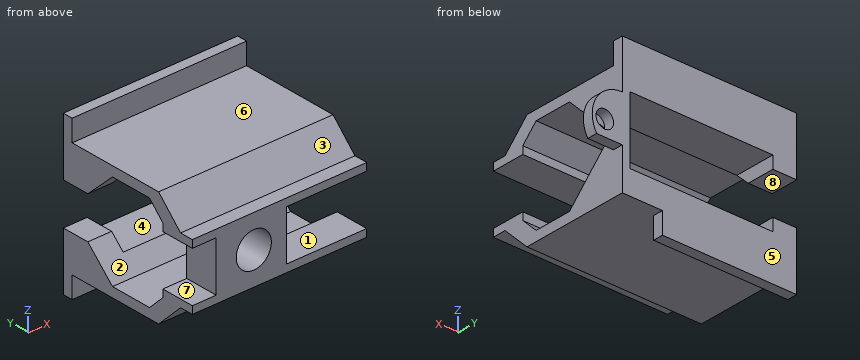
Autodesk Fusion 360 part; units mm, degrees
sketch "Sketch1" plane through (0, 0, 0) normal (0, 1, 0) x (1, 0, 0)
  line L0 (0, 0) -> (0, 11.5)
  line L1 (0, 0) -> (0, -8.3) construction
  line L2 (0, -8.3) -> (0, -19.8)
  line L3 (0, -19.8) -> (34.75, -19.8)
  line L4 (34.75, -19.8) -> (34.75, -10.025)
  line L5 (0, 11.5) -> (26.75, 11.5)
  line L6 (26.75, 11.5) -> (26.75, 7.25)
  line L7 (26.75, 7.25) -> (34.75, 7.25)
  line L8 (34.75, 7.25) -> (34.75, 1.85)
  line L9 (0, 0) -> (4.75, 0)
  line L10 (0, -8.3) -> (4.75, -8.3)
  line L11 (4.75, 0) -> (4.75, 2.475)
  line L12 (4.75, 2.475) -> (33.25, 2.475)
  line L13 (4.75, -8.3) -> (4.75, -10.775)
  line L14 (4.75, -10.775) -> (33.25, -10.775)
  line L15 (33.25, -10.775) -> (33.25, 2.475)
  line L16 (33.25, -4.15) -> (34.75, -4.15)
  arc A0 (34.75, -10.15) -> (34.75, 1.85) centre (34.75, -4.15) ccw
  line L17 (33.25, -4.15) -> (38.25, -4.15)
  circle A1 centre (38.25, -4.15) radius 1.75
  dimension "d1" = 11.5
  dimension "d2" = 8.3
  dimension "d3" = 11.5
  dimension "d4" = 34.75
  dimension "d5" = 9.775
  dimension "d6" = 26.75
  dimension "d7" = 4.25
  dimension "d8" = 8
  dimension "d10" = 4.75
  dimension "d11" = 4.75
  dimension "d12" = 2.475
  dimension "d13" = 28.5
  dimension "d14" = 2.475
  dimension "d15" = 28.5
  dimension "d16" = 12
  dimension "d17" = 5
  dimension "d18" = 3.5
extrude "Extrude1" add sketch "Sketch1" against normal blind 2
sketch "Sketch2" plane through (0, 0, 0) normal (-1, 0, 0) x (0, 0, 1)
  line L0 (0, 0) -> (-11.5, 0)
  line L1 (-11.5, 0) -> (-11.5, -2)
  line L2 (-11.5, -2) -> (0, -2)
  line L3 (0, -2) -> (0, 0)
  line L4 (0, -2) -> (0, -5.535)
  line L5 (8.3, -2) -> (8.3, -5.535)
  line L6 (0, -2) -> (-7.25, -2) construction
  line L7 (8.3, -2) -> (15.55, -2) construction
  line L8 (-7.25, -2) -> (-7.25, -21.5)
  line L9 (15.55, -2) -> (15.55, -21.5)
  line L10 (-7.25, -21.5) -> (-2.3003, -26.4497)
  line L11 (-7.25, -21.5) -> (-0.25, -21.5) construction
  line L12 (15.55, -21.5) -> (10.6003, -26.4497)
  line L13 (15.55, -21.5) -> (22.55, -21.5) construction
  line L14 (-2.3003, -26.4497) -> (-2.3003, -29.5997)
  line L15 (10.6003, -26.4497) -> (10.6003, -29.5997)
  line L16 (-2.3003, -29.5997) -> (10.6003, -29.5997)
  line L17 (-2.3003, -29.5997) -> (-2.3003, -22.4497) construction
  line L18 (10.6003, -29.5997) -> (10.6003, -22.4497) construction
  line L19 (10.6003, -22.4497) -> (-2.3003, -22.4497)
  line L20 (-2.3003, -22.4497) -> (-5.3055, -19.4445)
  line L21 (-2.3003, -22.4497) -> (1.9497, -22.4497) construction
  line L22 (10.6003, -22.4497) -> (13.6055, -19.4445)
  line L23 (10.6003, -22.4497) -> (14.8503, -22.4497) construction
  line L24 (-5.3055, -19.4445) -> (-5.3055, -11.0945)
  line L25 (13.6055, -19.4445) -> (13.6055, -11.0945)
  line L26 (-5.3055, -11.0945) -> (0, -5.535)
  line L27 (13.6055, -11.0945) -> (8.3, -5.535)
  line L28 (-7.25, -2) -> (0, -2)
  line L29 (8.3, -2) -> (15.55, -2)
  point P0 (8.3, -2)
  dimension "d24" = 3.535
  dimension "d25" = 3.535
  dimension "d26" = 7.25
  dimension "d27" = 7.25
  dimension "d28" = 19.5
  dimension "d29" = 19.5
  dimension "d30" = 45
  dimension "d31" = 7
  dimension "d32" = 135
  dimension "d33" = 7
  dimension "d34" = 3.15
  dimension "d35" = 3.15
  dimension "d36" = 7.15
  dimension "d37" = 7.15
  dimension "d38" = 135
  dimension "d39" = 4.25
  dimension "d40" = 45
  dimension "d41" = 4.25
  dimension "d42" = 8.35
  dimension "d43" = 8.35
extrude "Extrude2" add sketch "Sketch2" against normal blind 34.75 contours L2 L4 L5 L8 L9 L10 L12 L14 L15 L16 L19 L20 L22 L24 L25 L26 L27 L28 L29
extrude "Extrude3" cut 2 faces at (14.25, -2, -1.65) (23.75, -2, 9.125) along direction (0, -1, 0) blind 10
sketch "Sketch3" plane through (0, 0, 0) normal (0, 1, 0) x (-1, 0, 0)
  circle A0 centre (-38.25, 4.15) radius 1.75
  line L0 (0, 8.3) -> (0, 19.8)
  line L1 (0, 19.8) -> (-34.75, 19.8)
  line L2 (-34.75, 19.8) -> (-34.75, 10.15)
  arc A1 (-34.75, 10.15) -> (-34.75, -1.85) centre (-34.75, 4.15) ccw
  line L3 (-34.75, -1.85) -> (-34.75, -7.25)
  line L4 (-34.75, -7.25) -> (-26.75, -7.25)
  line L5 (-26.75, -7.25) -> (-26.75, -11.5)
  line L6 (-26.75, -11.5) -> (0, -11.5)
  line L7 (0, -11.5) -> (0, 0)
  line L8 (0, 0) -> (-4.75, 0)
  line L9 (-4.75, 0) -> (-4.75, -2.475)
  line L10 (-4.75, -2.475) -> (-33.25, -2.475)
  line L11 (-33.25, -2.475) -> (-33.25, 10.775)
  line L12 (-33.25, 10.775) -> (-4.75, 10.775)
  line L13 (-4.75, 10.775) -> (-4.75, 8.3)
  line L14 (-4.75, 8.3) -> (0, 8.3)
  line L15 (-34.75, -1.85) -> (-34.75, 1.025)
  line L16 (-34.75, 1.025) -> (-41.4539, 1.025)
  dimension "d48" = 2.875
extrude "Extrude4" cut sketch "Sketch3" against normal blind 13 contours A1 L15 L16
sketch "Sketch4" plane through (34.75, 0, 0) normal (1, 0, 0) x (0, 0, -1)
  line L0 (0, -5.535) -> (5.3055, -11.0945)
  line L1 (5.3055, -11.0945) -> (5.3055, -19.4445)
  line L2 (5.3055, -19.4445) -> (2.3003, -22.4497)
  line L3 (2.3003, -22.4497) -> (-10.6003, -22.4497)
  line L4 (-10.6003, -22.4497) -> (-13.6055, -19.4445)
  line L5 (-13.6055, -19.4445) -> (-13.6055, -11.0945)
  line L6 (-13.6055, -11.0945) -> (-8.3, -5.535)
  line L7 (-8.3, -5.535) -> (-8.3, -2)
  line L8 (-8.3, -2) -> (-10.15, -2)
  line L9 (-10.15, -2) -> (-10.15, 0)
  line L10 (-10.15, 0) -> (-19.8, 0)
  line L11 (-19.8, 0) -> (-19.8, -2)
  line L12 (-19.8, -2) -> (-15.55, -2)
  line L13 (-15.55, -2) -> (-15.55, -21.5)
  line L14 (-15.55, -21.5) -> (-10.6003, -26.4497)
  line L15 (-10.6003, -26.4497) -> (-10.6003, -29.5997)
  line L16 (-10.6003, -29.5997) -> (2.3003, -29.5997)
  line L17 (2.3003, -29.5997) -> (2.3003, -26.4497)
  line L18 (2.3003, -26.4497) -> (7.25, -21.5)
  line L19 (7.25, -21.5) -> (7.25, 0)
  line L20 (7.25, 0) -> (-1.025, 0)
  line L21 (-1.025, 0) -> (-1.025, -2)
  line L22 (-1.025, -2) -> (0, -2)
  line L23 (0, -2) -> (0, -5.535)
  line L24 (-3.535, -2) -> (-3.6055, -1.9295)
  line L25 (0, -5.535) -> (10, -5.535) construction
  line L26 (-4.765, -2) -> (-4.6945, -1.9295)
  line L27 (-8.3, -5.535) -> (1.7, -5.535) construction
  line L28 (-16, -15) -> (-15.5, -15)
  line L29 (-13.6055, -11.0945) -> (-13.6055, -11.9295)
  line L30 (-13.6055, -11.9295) -> (6.3945, -11.9295) construction
  line L31 (5.3055, -11.0945) -> (5.3055, -11.9295)
  line L32 (5.3055, -11.9295) -> (25.3055, -11.9295) construction
  line L33 (-8.3, -5.535) -> (-8.3, -2)
  line L34 (-8.3, -2) -> (0, -2)
  line L35 (0, -2) -> (0, -5.535)
  line L36 (0, -5.535) -> (5.3055, -11.0945)
  line L37 (-13.6055, -11.9295) -> (-4.15, -2.4741)
  line L38 (-3.6759, -2) -> (-3.6055, -1.9295)
  line L39 (5.3055, -11.9295) -> (-4.15, -2.4741)
  line L40 (-4.6241, -2) -> (-4.6945, -1.9295)
  dimension "d51" = 135
  dimension "d53" = 45
  dimension "d55" = 0.835
  dimension "d56" = 45
  dimension "d58" = 0.835
  dimension "d59" = 135
extrude "Extrude5" add sketch "Sketch4" against normal blind 1.5 contours L0 L1 L5 L6 L7 L22 L23 L29 L31 L33 L34 L35 L36 L37 L39
sketch "Sketch5" plane through (0, -29.5997, 0) normal (0, -1, 0) x (1, 0, 0)
  line L0 (0, 10.6003) -> (0, -2.3003)
  line L1 (0, -2.3003) -> (34.75, -2.3003)
  line L2 (34.75, -2.3003) -> (34.75, 10.6003)
  line L3 (34.75, 10.6003) -> (0, 10.6003)
  line L4 (0, 4.15) -> (12.25, 4.15)
  circle A0 centre (12.25, 4.15) radius 3.5
  dimension "d63" = 12.25
  dimension "d65" = 7
extrude "Extrude6" cut sketch "Sketch5" against normal blind 13 contours A0
sketch "Sketch6" plane through (34.75, 0, 0) normal (1, 0, 0) x (0, 0, -1)
  line L0 (-1.025, -2) -> (-10.15, -2)
  line L1 (-10.15, -2) -> (-10.15, 0)
  line L2 (-10.15, 0) -> (-19.8, 0)
  line L3 (-19.8, 0) -> (-19.8, -2)
  line L4 (-19.8, -2) -> (-15.55, -2)
  line L5 (-15.55, -2) -> (-15.55, -21.5)
  line L6 (-15.55, -21.5) -> (-10.6003, -26.4497)
  line L7 (-10.6003, -26.4497) -> (-10.6003, -29.5997)
  line L8 (-10.6003, -29.5997) -> (2.3003, -29.5997)
  line L9 (2.3003, -29.5997) -> (2.3003, -26.4497)
  line L10 (2.3003, -26.4497) -> (7.25, -21.5)
  line L11 (7.25, -21.5) -> (7.25, 0)
  line L12 (7.25, 0) -> (-1.025, 0)
  line L13 (-1.025, 0) -> (-1.025, -2)
  line L14 (-13.6055, -11.9295) -> (-4.15, -2.4741)
  line L15 (-4.15, -2.4741) -> (5.3055, -11.9295)
  line L16 (5.3055, -11.9295) -> (5.3055, -19.4445)
  line L17 (5.3055, -19.4445) -> (2.3003, -22.4497)
  line L18 (2.3003, -22.4497) -> (-10.6003, -22.4497)
  line L19 (-10.6003, -22.4497) -> (-13.6055, -19.4445)
  line L20 (-13.6055, -19.4445) -> (-13.6055, -11.9295)
  line L21 (2.3003, -29.5997) -> (0.8003, -29.5997)
  line L22 (-10.6003, -29.5997) -> (-9.1003, -29.5997)
  line L23 (-9.1003, -29.5997) -> (-9.1003, -22.4494)
  line L24 (0.8003, -29.5997) -> (0.8003, -22.4497)
  dimension "d69" = 1.5
  dimension "d70" = 1.5
  dimension "d71" = 7.15
extrude "Extrude7" cut sketch "Sketch6" against normal blind 16 contours L8 L18 L23 L24
sketch "Sketch7" plane through (0, 0, 0) normal (-1, 0, 0) x (0, 0, 1)
  line L0 (0, 0) -> (-11.5, 0)
  line L1 (-11.5, 0) -> (-11.5, -2)
  line L2 (-11.5, -2) -> (-7.25, -2)
  line L3 (-7.25, -2) -> (-7.25, -21.5)
  line L4 (-7.25, -21.5) -> (-2.3003, -26.4497)
  line L5 (-2.3003, -26.4497) -> (-2.3003, -29.5997)
  line L6 (-2.3003, -29.5997) -> (10.6003, -29.5997)
  line L7 (10.6003, -29.5997) -> (10.6003, -26.4497)
  line L8 (10.6003, -26.4497) -> (15.55, -21.5)
  line L9 (15.55, -21.5) -> (15.55, -2)
  line L10 (15.55, -2) -> (19.8, -2)
  line L11 (19.8, -2) -> (19.8, 0)
  line L12 (19.8, 0) -> (8.3, 0)
  line L13 (8.3, 0) -> (8.3, -5.535)
  line L14 (8.3, -5.535) -> (13.6055, -11.0945)
  line L15 (13.6055, -11.0945) -> (13.6055, -19.4445)
  line L16 (13.6055, -19.4445) -> (10.6003, -22.4497)
  line L17 (10.6003, -22.4497) -> (-2.3003, -22.4497)
  line L18 (-2.3003, -22.4497) -> (-5.3055, -19.4445)
  line L19 (-5.3055, -19.4445) -> (-5.3055, -11.0945)
  line L20 (-5.3055, -11.0945) -> (0, -5.535)
  line L21 (0, -5.535) -> (0, 0)
  line L22 (10.6003, -29.5997) -> (9.1003, -29.5997)
  line L23 (-2.3003, -29.5997) -> (-0.8003, -29.5997)
  line L24 (-0.8003, -29.5997) -> (-0.8003, -22.4497)
  line L25 (9.1003, -29.5997) -> (9.1003, -22.4497)
  point P0 (-0.8003, -22.4497)
  point P1 (9.1003, -22.4497)
  dimension "d74" = 1.5
  dimension "d75" = 1.5
extrude "Extrude8" cut sketch "Sketch7" against normal blind 4.75 contours L6 L17 L24 L25
extrude "Extrude9" cut 1 faces at (6.0833, -29.5997, 4.15) along direction (0, 1, 0) blind 0.5
sketch "Sketch8" plane through (0, 0, 0) normal (0, 1, 0) x (-1, 0, 0)
  line L0 (-39.872, 1.025) -> (-34.75, 1.025)
  line L1 (-34.75, 1.025) -> (-34.75, -7.25)
  line L2 (-34.75, -7.25) -> (-26.75, -7.25)
  line L3 (-26.75, -7.25) -> (-26.75, -11.5)
  line L4 (-26.75, -11.5) -> (0, -11.5)
  line L5 (0, -11.5) -> (0, 0)
  line L6 (0, 0) -> (-4.75, 0)
  line L7 (-4.75, 0) -> (-4.75, -2.475)
  line L8 (-4.75, -2.475) -> (-33.25, -2.475)
  line L9 (-33.25, -2.475) -> (-33.25, 10.775)
  line L10 (-33.25, 10.775) -> (-4.75, 10.775)
  line L11 (-4.75, 10.775) -> (-4.75, 8.3)
  line L12 (-4.75, 8.3) -> (0, 8.3)
  line L13 (0, 8.3) -> (0, 19.8)
  line L14 (0, 19.8) -> (-34.75, 19.8)
  line L15 (-34.75, 19.8) -> (-34.75, 10.15)
  arc A0 (-34.75, 10.15) -> (-39.872, 1.025) centre (-34.75, 4.15) ccw
  circle A1 centre (-38.25, 4.15) radius 1.75
  line L16 (-34.75, 10.15) -> (-34.75, 1.025)
  line L17 (-34.75, 4.15) -> (-38.25, 4.15)
equation "d17 = HolePosX"
equation "d18 = HoleSize"
equation "HolePosX = 5 mm"
equation "HoleSize = 3.5 mm"
equation "TopThickness = 2 mm"
equation "d63 = JointPosX"
equation "JointPosX = 12.25 mm"
equation "d65 = HoleBall"
equation "HoleBall = 7 mm"
Can you work these out from the model? Positions are in its coordinate system, mm. Face numbers are marked on the shaded views. A direction names the side the tool comes from. Coordinates: 2 decimals unless noted, no trailing zeros. Write each loop counter-clockwise with the first axis right and the second up, starting at its lowest first coordinate (ties: lowest second). Pieces come first, ordered by that corner, then holes. Notation, with made-up numbers: (39.5, 50) -> (63.5, 50) arc R14 cw to (63.5, 72) -> close; hole circle Ø6 at (53.5, 48). An arc over 180 degrees is marked (long way). Write each question's results on one line, items separated by ' | '. Start each with the question number.
Q1. Imagine slicing it at C-C (y = -9). Write out the boundary of the cut face in (x, z), then the cut area to 3 significant figures.
Q2. Imagine slicing it at D-D (z = 12). Write out the boundary of the cut face in (x, y), then the cut area to 3 significant figures.
Q3. On a 3-axis mill with a long thin cutter (end or side, diameter ignored), from which of +Z, -Z, +X, -X, +Y, -Y can I reach the whole of each face in a straight line? I mean the marked faces 4, 5, 6, 7 and 8. Say none if no direction works.
Q4. If I drill on probe 1 along Z at (x, y) = (7, -12); probe 2 along Z at (x, y) = (21, -5.5) (3 decimals); probe 3 along X at (y, z) = (-0.65, 4.15), over which ranges is the centre line in solid material (lowest first)?
Q5. Imagine slicing it at A-A (y = -23.25). Write out the boundary of the cut face in (x, z), then the cut area to 3 significant figures.
Q6. I'm going to push flat-ended pins straight in: pin 1 (8 mm diameter, centred on y = -19.5, z = -4.5, fed in from +X); pin 2 (6.5 mm diameter, centred on x = 15.5, y = -16.5, fed in from +Z); pin 3 (2 mm diameter, centred on x = 26, z = 18.5, fed in from -Y). Where does each tip first touch, or does it pass through?
Q7. We'd pull the mould along Y, two halves only. Please class the marked faces 1, 2 and 3: +Y half, -Y half, draft (parallel to the pull), parting line (faces both ways), or undercut.
Taken from the geometry:
1) outline: (0, -7.25) -> (34.75, -7.25) -> (34.75, -2.38) -> (33.25, -2.38) -> (33.25, -3.31) -> (0, -3.31) -> close; (0, 11.61) -> (33.25, 11.61) -> (33.25, 10.68) -> (34.75, 10.68) -> (34.75, 15.55) -> (0, 15.55) -> close | area: 277 mm^2
2) outline: (0, -25.05) -> (34.75, -25.05) -> (34.75, -21.05) -> (0, -21.05) -> close; (0, -9.41) -> (33.25, -9.41) -> (33.25, -10.32) -> (34.75, -10.32) -> (34.75, 0) -> (0, 0) -> close | area: 467 mm^2
3) face 4: +Y | face 5: +Z, -Z, +X, -X, +Y | face 6: +Z, +X, -X, -Y | face 7: -X, -Y | face 8: -X, +Y, -Y
4) probe 1: z = -7.25 to -5.31, 13.61 to 15.55 | probe 2: z = -7.25 to -2.475, 10.775 to 15.55 | probe 3: x = 33.25 to 36.5, 40 to 40.75
5) outline: (0, -5.5) -> (34.75, -5.5) -> (34.75, -0.8) -> (18.75, -0.8) -> (18.75, 9.1) -> (34.75, 9.1) -> (34.75, 13.8) -> (0, 13.8) -> (0, 9.1) -> (4.75, 9.1) -> (4.75, -0.8) -> (0, -0.8) -> close; hole circle Ø7 at (12.25, 4.15) | area: 427 mm^2
6) pin 1: stops at x = 34.75 | pin 2: stops at z = 15.55 | pin 3: stops at y = -2
7) face 1: draft | face 2: undercut | face 3: -Y half
